The model under review builds one solid part; all positions refer to its coordinate system, in mm. A direction names the side the tool comes from. Round coordinates to 2 decimals unless told otherwise and drop trailing zeros. Loops run counter-clockwise (first coordinate to the right, second up) from the corner with the lowest first, then second, coordinate; pieces in that order, holes last. Notation, with made-up numbers: (7.25, 30) -> (60.25, 30) arc R25 ccw to (60.25, 68) -> close; hole circle Ø4 at (28, 65.5). An arc over 180 degrees is marked (long way). Write each question's results on one line, items separated by ' | '. Start each with the question number.
Item 1: We need section A-A (x = 20). Give the boundary of the cut face in (y, z).
Item 2: For L1, parallel to X at y = -16, z = 6; L2, parallel to Y at x = 175, z = 7; L3, parallel to X at y = -22, z = 4.75, list the stretches that pass through material, from the lowest coordinate up. Write a range as from..to.
Item 3: Mouldability with a two-part tool opening along X and no side actions: class faces 1 (the flat face through (0, -13, 4)), 2 (the flat face through (125, 0, 4)), 3 (the flat face through (246.38, -19, 4)), 4 (the flat face through (254, -8, 4)) as pulls with the +X half, pulls with the -X half, needs draft (parallel to the pull), parting line crosses it, or undercut.
Item 4: We need section B-B (y = -21). Give the boundary of the cut face in (x, z).
Item 5: Tool access review of faces 5 (the flat face through (125, -7, 6.35)), 6 (the flat face through (250, -23.324, 4)), 7 (the flat face through (125, -13, 0)): name each direction out of +Z, -Z, +X, -X, +Y, -Y from which nothing blocks a thin tool from reaching the whole face with its end or side.
Autodesk Inventor part; units mm, degrees
ref_plane "YZ Plane" through (0, 0, 0) normal (1, 0, 0) x (0, 1, 0)
ref_plane "XZ Plane" through (0, 0, 0) normal (0, 1, 0) x (-1, 0, 0)
ref_plane "XY Plane" through (0, 0, 0) normal (0, 0, 1) x (1, 0, 0)
sketch "Sketch1" plane through (0, 0, 0) normal (0, 0, 1) x (1, 0, 0)
  line L0 (0, 0) -> (254, 0)
  line L1 (254, 0) -> (254, -25.4)
  line L2 (254, -25.4) -> (0, -25.4)
  line L3 (0, -25.4) -> (0, 0)
  dimension "d0" = 254
  dimension "d1" = 25.4
extrude "Extrusion1" add sketch "Sketch1" along normal blind 7.62
sketch "Sketch2" plane through (0, 0, 7.62) normal (0, 0, 1) x (1, 0, 0)
  line L0 (0, -25.4) -> (0, 0)
  line L1 (0, -3.7895) -> (254, -3.7895)
  line L2 (254, -3.7895) -> (254, -10.1395)
  line L3 (254, -10.1395) -> (0, -10.1395)
  line L4 (0, -10.1395) -> (0, -3.7895)
  dimension "d4" = 254
  dimension "d5" = 6.35
extrude "Extrusion2" cut sketch "Sketch2" against normal blind 1.27
sketch "Sketch3" plane through (254, -25.4, 0) normal (1, 0, 0) x (0, 0, -1)
  line L0 (-7.62, 15.2605) -> (-7.62, 0)
  line L1 (-7.62, 2.0757) -> (0, 2.0757)
  line L2 (0, 2.0757) -> (0, 9.6957)
  line L3 (0, 9.6957) -> (-7.62, 9.6957)
  line L4 (-7.62, 9.6957) -> (-7.62, 2.0757)
  dimension "d8" = 7.62
  dimension "d9" = 7.62
extrude "Extrusion3" cut sketch "Sketch3" against normal blind 7.62
sketch "Sketch4" plane through (254, -23.3243, 7.62) normal (0, 1, 0) x (1, 0, 0)
  circle A0 centre (-3.2098, 1.884) radius 1.27
  circle A1 centre (-3.1463, 5.6104) radius 1.27
  point P0 (-254, 7.62)
extrude "Extrusion4" add sketch "Sketch4" along normal blind 7.62
properties part number "Bar"
Here are the results:
1) outline: (-25.4, 0) -> (0, 0) -> (0, 7.62) -> (-3.79, 7.62) -> (-3.79, 6.35) -> (-10.14, 6.35) -> (-10.14, 7.62) -> (-25.4, 7.62) -> close
2) L1: x = 0..246.38, 249.55..252.03 | L2: y = -25.4..-10.14, -3.79..0 | L3: x = 0..246.38, 249.99..251.59
3) face 1: pulls with the -X half | face 2: needs draft | face 3: undercut | face 4: pulls with the +X half
4) outline: (0, 0) -> (246.38, 0) -> (246.38, 7.62) -> (0, 7.62) -> close; circle Ø2.54 at (250.79, 5.74); circle Ø2.54 at (250.85, 2.01)
5) face 5: +Z, +X, -X | face 6: none | face 7: -Z, +X, -X, +Y, -Y
